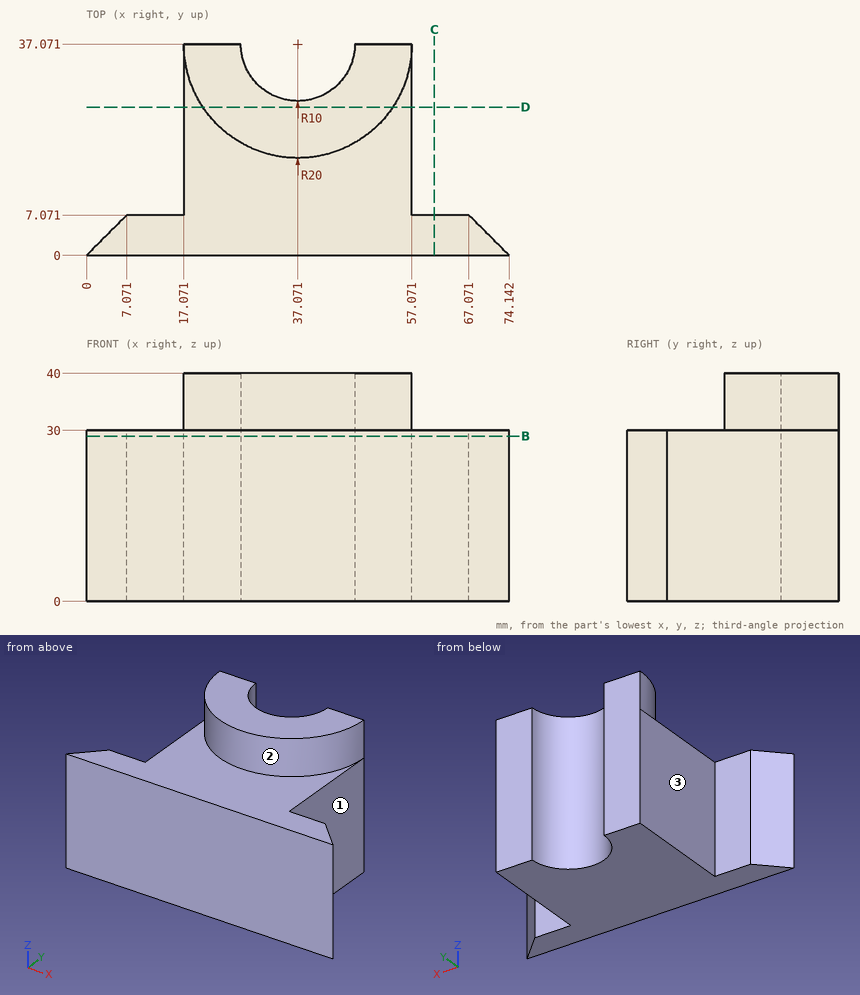
Source: three-view drawing plus pictorial views. Frame: mm from the lowest corner of the part. A direction names the side the tool comes from. Round coordinates to 2 decimals unless told otherwise and drop trailing zeros. Loops run counter-clockwise (first coordinate to the right, second up) from the corner with the lowest first, then second, coordinate; pieces in that order, holes last.
Q1. Pin query (flat end, axial travel): P1, Ø3, axis at x = 11, z = 9.5, coming from the -Y side; P2, Ø3, axis at x = 10.5, z = 18, coming from the +Y side; P3, Ø10, axis at y = 30.5, z = 29, coming from the +X side; P4, Ø8, axis at x = 10.5, y = 5, coming from the +Z side. Return the tip coordinate at first contact, or that it passes through.
Q2. Section B-B on z = 29. Return loops of the section in (x, y), plus the area to 3 significant figures.
Q3. Section D-D on y = 26. Return loops of the section in (x, z) (1 decimal).
Q4. Material intervals for L1, parallel to Z at x = 48, y = 12; L2, parallel to X at y = 10, z = 12.5; L3, parallel to X at y = 30.5, z = 17.5, sorted ascending.
Q5. Access query for the marked faces 1, 2 and 3. Directions: +Z, -Z, +X, -X, +Y, -Y. A direction counts if a zero-diameter tool reaches every point of the face in a straight line with its end or side. Return the directions, or none.
Q6. Section C-C on x = 61. Return loops of the section in (y, z), plus the area to 3 significant figures.
Evaluation:
1. P1: stops at y = 0
1. P2: stops at y = 7.07
1. P3: stops at x = 57.07
1. P4: stops at z = 30
2. outline: (0, 0) - (74.14, 0) - (67.07, 7.07) - (57.07, 7.07) - (57.07, 37.07) - (47.07, 37.07) arc R10 cw to (27.07, 37.07) - (17.07, 37.07) - (17.07, 7.07) - (7.07, 7.07) - close
2. area: 1,520 mm2
3. outline: (17.1, 0) - (57.1, 0) - (57.1, 30) - (53.7, 30) - (53.7, 40) - (20.4, 40) - (20.4, 30) - (17.1, 30) - close
4. L1: z = 0 to 30
4. L2: x = 17.07 to 57.07
4. L3: x = 17.07 to 29.53, 44.61 to 57.07
5. face 1: +Z, -Z, +X, +Y
5. face 2: +Z, -Y
5. face 3: +Z, -Z, -X, +Y
6. outline: (0, 0) - (7.07, 0) - (7.07, 30) - (0, 30) - close
6. area: 212 mm2
